from build123d import *

# Parameters (mm, degrees)
SKETCH1_W                      = 100
SKETCH1_H                      = 30
SKETCH1_R                      = 1.625
BOSS_EXTRUDE1_DEPTH            = 6
FILLET1_R                      = 15
CBORE_FOR_M2_SHCS1_D           = 2.4
CBORE_FOR_M2_SHCS1_DEPTH       = 20
CBORE_FOR_M2_SHCS1_CBORE_D     = 4.4
CBORE_FOR_M2_SHCS1_CBORE_DEPTH = 2
CBORE_FOR_M2_SHCS1_TIP         = 0.721032743


with BuildPart() as part:
    # Sketch1 → Boss-Extrude1 (new body)
    with BuildSketch(Plane(origin=(0, 0, 0), x_dir=(0, 0, -1), z_dir=(1, 0, 0))):
        Rectangle(SKETCH1_W, SKETCH1_H)
        with Locations((-30, 5)):
            Circle(SKETCH1_R, mode=Mode.SUBTRACT)
    extrude(amount=BOSS_EXTRUDE1_DEPTH)

    # Fillet1
    fillet1_edges = [part.edges().sort_by_distance(p)[0] for p in [
        (3, -15, 50),
    ]]
    fillet(fillet1_edges, radius=FILLET1_R)

    # CBORE for M2 SHCS1
    with Locations(Plane(origin=(-622.293536786, 25, -1323.282701689), x_dir=(1, 0, 0), z_dir=(0, 1, 0))):
        with Locations((727.293536786, -1277.282701689), (727.293536786, -1361.282701689), (625.293536786, -1277.282701689), (625.293536786, -1361.282701689), (625.293536786, -1319.282701689), (727.293536786, -1319.282701689)):
            CounterBoreHole(CBORE_FOR_M2_SHCS1_D / 2, CBORE_FOR_M2_SHCS1_CBORE_D / 2, CBORE_FOR_M2_SHCS1_CBORE_DEPTH, depth=CBORE_FOR_M2_SHCS1_DEPTH)
            with Locations((0, 0, -(CBORE_FOR_M2_SHCS1_DEPTH + CBORE_FOR_M2_SHCS1_TIP / 2))):  # 118° drill point
                Cone(0, CBORE_FOR_M2_SHCS1_D / 2, CBORE_FOR_M2_SHCS1_TIP, mode=Mode.SUBTRACT)


solid = part.part
Could you check a few things on this model? Use its own coordinates, in mm. A direction names the side the tool comes from. Round coordinates to 2 decimals unless told otherwise and drop trailing zeros. Write each loop counter-clockwise with the first axis right and the second up, starting at its lowest first coordinate (ties: lowest second). Pieces come first, ordered by that corner, then holes. Notation, with made-up numbers: (-9.75, 49) - (0.25, 49) arc R10 ccw to (0.25, 61) - close; hole circle Ø2 at (10, 26.5). An arc over 180 degrees is marked (long way). Put each result on its own line as item: value. Start each with the question number.
(1) I want a section at B-B, the plane z = 30. Please give me the cut outline in (x, y) (3 decimals), plus the area to 4 significant figures.
(2) I want a section at A-A, the plane y = 11.5. Please give me the cut outline in (x, z).
(3) For faces 5 (the flat face through (3, 0, -50)), 6 (the cylindrical face through (3.16, 9.93, -5.19)), which set-ups out of +Z, -Z, +X, -X, +Y, -Y let a thin tool reach every point of the face, with its end or its side?
(4) Thinking about a two-plate mould opening in Z: for faces 1 (the cylindrical face through (3.16, 9.93, -47.19)), 2 (the cylindrical face through (2.958, 5.071, 31.623)), 3 (the flat face through (0, 0, 1)), 4 (the flat face through (3, 7, 50)), which applies, released by +Z, released by -Z, zero draft, split by the parting line, or undercut?
(5) Will this pin go through, and if not, where does the flat tip stop? pin 1 (1.9 mm diameter, centred on x = 3, z = -4, fed in from +Y).
(6) I need wall thicknesses on probe 1 along Z at (x, y) = (3, 12); probe 2 along Y at (x, z) = (4.85, 30) (3 decimals); probe 3 along Z at (x, y) = (2.15, 14). Which ranges of each line are inside material? Lowest first, please.
(7) I want a section at C-C, the plane z = 42. Please give me the cut outline in (x, y), plus the area to 3 significant figures.
Here are the results:
1. outline: (0, -15) - (6, -15) - (6, 3.375) - (0, 3.375) - close; (0, 6.625) - (6, 6.625) - (6, 15) - (0, 15) - close
1. area: 160.5 mm^2
2. outline: (0, -50) - (6, -50) - (6, 50) - (0, 50) - close; hole circle Ø2.4 at (3, -46); hole circle Ø2.4 at (3, -4); hole circle Ø2.4 at (3, 38)
3. face 5: -Z, +X, -X, +Y, -Y
3. face 6: +Y
4. face 1: undercut
4. face 2: undercut
4. face 3: zero draft
4. face 4: released by +Z
5. pin 1: stops at y = 4.85
6. probe 1: z = -50 to -47.2, -44.8 to -5.2, -2.8 to 36.8, 39.2 to 50
6. probe 2: y = -15 to 3.375, 6.625 to 15
6. probe 3: z = -50 to -46.85, -45.15 to -4.85, -3.15 to 37.15, 38.85 to 50
7. outline: (0, -13.27) - (6, -13.27) - (6, 15) - (0, 15) - close
7. area: 170 mm^2
